from build123d import *

# Parameters (mm, degrees)
BOSS_EXTRUDE2_START = -20
SKETCH3_R           = 4.25
BOSS_EXTRUDE2_DEPTH = 30
BOSS_EXTRUDE3_START = 10
SKETCH4_R           = 8.5
BOSS_EXTRUDE3_DEPTH = 10
SKETCH5_W           = 17
SKETCH5_H           = 42
BOSS_EXTRUDE4_DEPTH = 10
SKETCH6_R           = 8.5
BOSS_EXTRUDE5_DEPTH = 20
SKETCH9_W           = 7
SKETCH9_H           = 7
CUT_EXTRUDE1_DEPTH  = 20
BOSS_EXTRUDE7_DEPTH = 10
BOSS_EXTRUDE8_DEPTH = 20


with BuildPart() as part:
    # Sketch3 → Boss-Extrude2 (new body)
    with BuildSketch(Plane.XY.offset(16).offset(BOSS_EXTRUDE2_START)):
        Circle(SKETCH3_R)
    extrude(amount=BOSS_EXTRUDE2_DEPTH)



with BuildPart() as body_2:
    # Sketch4 → Boss-Extrude3 (new body)
    with BuildSketch(Plane(origin=(0, 0, -4), x_dir=(-1, 0, 0), z_dir=(0, 0, -1)).offset(BOSS_EXTRUDE3_START)):
        Circle(SKETCH4_R)
    extrude(amount=BOSS_EXTRUDE3_DEPTH)

    # Sketch5 → Boss-Extrude4 (add)
    with BuildSketch(Plane(origin=(0, 0, -24), x_dir=(-1, 0, 0), z_dir=(0, 0, -1))):
        with Locations((0, -12.5)):
            Rectangle(SKETCH5_W, SKETCH5_H)
    extrude(amount=-BOSS_EXTRUDE4_DEPTH)

    # Sketch6 → Boss-Extrude5 (add)
    with BuildSketch(Plane(origin=(0, 0, -24), x_dir=(-1, 0, 0), z_dir=(0, 0, -1))):
        with Locations((0, -25)):
            Circle(SKETCH6_R)
    extrude(amount=BOSS_EXTRUDE5_DEPTH)

    # Sketch9 → Cut-Extrude1 (cut)
    with BuildSketch(Plane(origin=(0, 0, -44), x_dir=(-1, 0, 0), z_dir=(0, 0, -1))):
        with Locations((0, -25)):
            Rectangle(SKETCH9_W, SKETCH9_H)
    extrude(amount=-CUT_EXTRUDE1_DEPTH, mode=Mode.SUBTRACT)


with BuildPart() as part_1:
    add(part.part)

    add(body_2.part)  # Boss-Extrude7 merges body 2
    # Sketch11 → Boss-Extrude7 (add)
    with BuildSketch(Plane.XY.offset(-14)):
        with BuildLine():
            Line((3.4, -7.681145748), (3.4, -11.4))
            Line((3.4, -11.4), (-3.4, -11.4))
            Line((-3.4, -11.4), (-3.4, -7.681145748))
            ThreePointArc((-3.4, -7.681145748), (-8.4, 0), (-3.4, 7.681145748))
            Line((-3.4, 7.681145748), (-3.4, 11.4))
            Line((-3.4, 11.4), (3.4, 11.4))
            Line((3.4, 11.4), (3.4, 7.681145748))
            ThreePointArc((3.4, 7.681145748), (8.4, 0), (3.4, -7.681145748))
        make_face()
    extrude(amount=BOSS_EXTRUDE7_DEPTH)

    # Sketch13 → Boss-Extrude8 (add)
    with BuildSketch(Plane.XY.offset(26)):
        with BuildLine():
            Line((-1.949358869, 1.4), (-3.906724971, 1.4))
            ThreePointArc((-3.906724971, 1.4), (-4.15, 0), (-3.906724971, -1.4))
            Line((-3.906724971, -1.4), (-1.949358869, -1.4))
            ThreePointArc((-1.949358869, -1.4), (0, -2.4), (1.949358869, -1.4))
            Line((1.949358869, -1.4), (3.906724971, -1.4))
            ThreePointArc((3.906724971, -1.4), (4.15, 0), (3.906724971, 1.4))
            Line((3.906724971, 1.4), (1.949358869, 1.4))
            ThreePointArc((1.949358869, 1.4), (0, 2.4), (-1.949358869, 1.4))
        make_face()
    extrude(amount=BOSS_EXTRUDE8_DEPTH)


solid = part_1.part
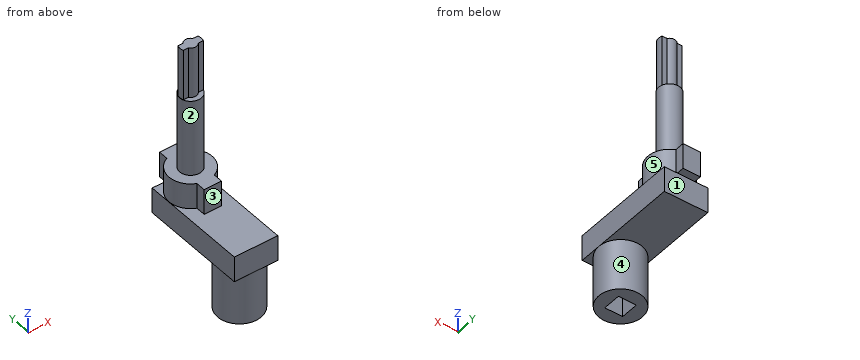
Here's how the part is built. I have some questions about the finished solid (model axes, mm). Face numbers are marked on the shaded views. A direction names the side the tool comes from. Coordinates: 2 decimals unless noted, no trailing zeros. Write each loop counter-clockwise with the first axis right and the second up, starting at its lowest first coordinate (ties: lowest second). Pieces come first, ordered by that corner, then holes.
Item 1: Will these pins go through, and if not, where does the flat tip stop? pin 1 (2 mm diameter, centred on x = 2.5, z = 38, fed in from +Y); pin 2 (5 mm diameter, centred on x = -5.5, y = -20.5, fed in from +Z); pin 3 (1.9 mm diameter, centred on y = 10, z = -6.5, fed in from -X).
Item 2: I want a section at C-C on x = 6. Write out the boundary of the cut face in (y, z).
Item 3: On a 3-axis mill with a long thin cutter (end or side, diameter ignored), from which of +Z, -Z, +X, -X, +Y, -Y can I reach the whole of each face in a straight line? I mean the marked faces 1, 2, 3, 4 and 5. Say none if no direction works.
Item 4: I want a section at B-B on z = 30. Write out the boundary of the cut face in (x, y), and give its area (3 significant figures).
Item 5: If I drill on line 1 (Z direction, x = 3.75, y = -27); line 2 (Z direction, x = -1.75, y = 2.5); line 3 (Y direction, x = -3.75, z = -18), over which ranges is the centre line in solid material (lowest first)?
Item 6: I want a section at A-A on y = 0. Write out the boundary of the cut face in (x, z), and give its area (3 significant figures).
Item 7: I want a section at D-D on z = 9.5. Write out the boundary of the cut face in (x, y).
Findings below:
1. pin 1: stops at y = 1.87
1. pin 2: stops at z = -14
1. pin 3: stops at x = -3.4
2. outline: (-33.5, -24) - (-31.02, -24) - (-31.02, -44) - (-18.98, -44) - (-18.98, -24) - (8.5, -24) - (8.5, -14) - (5.88, -14) - (5.88, -4) - (-5.88, -4) - (-5.88, -14) - (-33.5, -14) - close
3. face 1: -Z, +X, -X, +Y
3. face 2: +Z
3. face 3: +Z, +X, -X, -Y
3. face 4: -Z
3. face 5: +Z, +X
4. outline: (-3.91, -1.4) - (-1.95, -1.4) arc R2.4 ccw to (1.95, -1.4) - (3.91, -1.4) arc R4.15 ccw to (3.91, 1.4) - (1.95, 1.4) arc R2.4 ccw to (-1.95, 1.4) - (-3.91, 1.4) arc R4.15 ccw to start
4. area: 28.3 mm2
5. line 1: z = -44 to -14
5. line 2: z = -24 to 26
5. line 3: y = -33.5 to 8.5
6. outline: (-8.5, -24) - (8.5, -24) - (8.5, -14) - (8.4, -14) - (8.4, -4) - (4.25, -4) - (4.25, 26) - (4.15, 26) - (4.15, 46) - (-4.15, 46) - (-4.15, 26) - (-4.25, 26) - (-4.25, -4) - (-8.4, -4) - (-8.4, -14) - (-8.5, -14) - close
6. area: 759 mm2
7. outline: circle Ø8.5 at (0, 0)
